Input: part model. Units: mm. Frame: model coordinates. A direction names the side the tool comes from. Give positions to 0.01 mm unless a question says otherwise; leave off trailing zeros. Order: outer loops, then holes, each group sorted by start corner. A loop starts at its lowest first (then second) coordinate and runs counter-clockwise, first axis right, second up. Notation, with made-up numbers: (83.5, -11.75) - (99.5, -11.75) arc R11 cw to (99.5, -1.75) - close; hole circle Ø4 at (54.5, 42.5). An arc over 180 degrees is marked (long way). Use a Markdown table: item, result.
from build123d import *

# Parameters (mm, degrees)
SKETCH_1_R      = 1.6
EXTRUDE_1_DEPTH = 3
FILLET_1_R      = 5
FILLET_2_R      = 1


with BuildPart() as part:
    # 草图1 → 凸台-拉伸1 (new body)
    with BuildSketch(Plane(origin=(0, 0, 0), x_dir=(1, 0, 0), z_dir=(0, 1, 0))):
        Polygon((8, -26), (8, -8), (16, -8), (16, -26), (46, -26), (46, 26), (-46, 26), (-46, -26), align=None)
        with Locations(Location((-36, 16, 0), (0, 0, 270))):
            Circle(SKETCH_1_R, mode=Mode.SUBTRACT)
        with Locations(Location((-36, -16, 0), (0, 0, 270))):
            Circle(SKETCH_1_R, mode=Mode.SUBTRACT)
        with Locations(Location((36, -16, 0), (0, 0, 270))):
            Circle(SKETCH_1_R, mode=Mode.SUBTRACT)
        with Locations(Location((36, 16, 0), (0, 0, 270))):
            Circle(SKETCH_1_R, mode=Mode.SUBTRACT)
    extrude(amount=EXTRUDE_1_DEPTH)

    # 圆角1
    fillet_1_edges = [part.edges().sort_by_distance(p)[0] for p in [
        (-46, 1.5, 26),
        (-46, 1.5, -26),
        (46, 1.5, -26),
        (46, 1.5, 26),
    ]]
    fillet(fillet_1_edges, radius=FILLET_1_R)

    # 圆角2
    fillet_2_edges = [part.edges().sort_by_distance(p)[0] for p in [
        (16, 1.5, 26),
        (16, 1.5, 8),
        (8, 1.5, 8),
        (8, 1.5, 26),
    ]]
    fillet(fillet_2_edges, radius=FILLET_2_R)


solid = part.part
1. Section query C-C (x = 36). Return loops of the section in (y, z), then the cut area to 3 significant figures.
Response:
| item | result |
|---|---|
| outline | (0, -26) - (3, -26) - (3, -17.6) - (0, -17.6) - close; (0, -14.4) - (3, -14.4) - (3, 14.4) - (0, 14.4) - close; (0, 17.6) - (3, 17.6) - (3, 26) - (0, 26) - close |
| area | 137 mm^2 |
2. Section query A-A (z = 16). Return loops of the section in (x, y).
Response:
| item | result |
|---|---|
| outline | (-46, 0) - (-37.6, 0) - (-37.6, 3) - (-46, 3) - close; (-34.4, 0) - (8, 0) - (8, 3) - (-34.4, 3) - close; (16, 0) - (34.4, 0) - (34.4, 3) - (16, 3) - close; (37.6, 0) - (46, 0) - (46, 3) - (37.6, 3) - close |
3. Section query B-B (z = -16). Return loops of the section in (x, y), then the cut area to 3 significant figures.
Response:
| item | result |
|---|---|
| outline | (-46, 0) - (-37.6, 0) - (-37.6, 3) - (-46, 3) - close; (-34.4, 0) - (34.4, 0) - (34.4, 3) - (-34.4, 3) - close; (37.6, 0) - (46, 0) - (46, 3) - (37.6, 3) - close |
| area | 257 mm^2 |
4. Section query D-D (y = 0.9). Return loops of the section in (x, z).
Response:
| item | result |
|---|---|
| outline | (-46, -21) arc R5 ccw to (-41, -26) - (41, -26) arc R5 ccw to (46, -21) - (46, 21) arc R5 ccw to (41, 26) - (17, 26) arc R1 ccw to (16, 25) - (16, 9) arc R1 cw to (15, 8) - (9, 8) arc R1 cw to (8, 9) - (8, 25) arc R1 ccw to (7, 26) - (-41, 26) arc R5 ccw to (-46, 21) - close; hole circle Ø3.2 at (-36, -16); hole circle Ø3.2 at (-36, 16); hole circle Ø3.2 at (36, -16); hole circle Ø3.2 at (36, 16) |
5. Pin query (flat end, axial travel): pin 1 (2.5 mm diameter, centred on x = -36, z = -16, fed in from +Y); pin 2 (6 mm diameter, centred on x = 36, z = -20, fed in from -Y). Return the tip coordinate at first contact, or that it passes through.
Response:
| item | result |
|---|---|
| pin 1 | passes through |
| pin 2 | stops at y = 0 |
6. Set-up query: faces 1 (the face through (29, 1, 26)), 2 (the face through (16, 1, 17)). Return all of +Z, -Z, +X, -X, +Y, -Y with unobstructed straight access to the full face (end or side cutting, diameter ignored); none if empty.
Response:
| item | result |
|---|---|
| face 1 | +Z, +X, -X, +Y, -Y |
| face 2 | +Z, +Y, -Y |
7. Mould query, pull axis X, two halves, no side actions, for faces 3 (the face through (8, 1, 17)), 4 (the face through (12, 1, 8)), 5 (the face through (44, 2, -25)), 6 (the face through (-44, 2, 25)). Classes: pulls with the +X half, pulls with the -X half, needs draft (parallel to the pull), parting line crosses it, or undercut.
Response:
| item | result |
|---|---|
| face 3 | undercut |
| face 4 | undercut |
| face 5 | pulls with the +X half |
| face 6 | pulls with the -X half |
8. Material intervals for line 1 along X through (y, z) = (0.8, -16); line 2 along X through (y, z) = (0.9, 16); line 3 along X through (y, z) = (1.8, 14), sorted ascending.
Response:
| item | result |
|---|---|
| line 1 | x = -46 to -37.6, -34.4 to 34.4, 37.6 to 46 |
| line 2 | x = -46 to -37.6, -34.4 to 8, 16 to 34.4, 37.6 to 46 |
| line 3 | x = -46 to 8, 16 to 46 |
